Answer from the drawing. Dimensions are ordinates in mm from the lowest x, y and z of the part. A direction names the side the tool comes from. Give positions to 0.01 mm unless a question says otherwise; leave off trailing zeros. Loops run counter-clockwise (first coordinate to the right, second up) from the corner with the lowest first, then second, coordinate; pieces in that order, holes last. Notation, with made-up numbers: (4, -37.75) - (33, -37.75) arc R13 ccw to (33, -18.75) - close; hole circle Ø4 at (14, -35). An arc over 180 degrees is marked (long way). Put each result on its own line as item: value. Start each with the question number.
1. A cutting plane is placed at B-B, the plane y = 46.5. Determine the outline of the cut face in (x, z) (3 decimals), plus the area to 3 significant figures.
2. A cutting plane is placed at C-C, the plane z = 7. Determine the outline of the cut face in (x, y) (3 decimals).
3. A cutting plane is placed at A-A, the plane x = 41. Determine the outline of the cut face in (y, z), plus the area to 3 significant figures.
4. A cutting plane is placed at D-D, the plane x = 18.5. Determine the outline of the cut face in (y, z), plus the area to 3 significant figures.
5. For a pull along X with two mould halves and no side action, classify the marked faces 1, 2 and 3 as released by +X, released by -X, zero draft, split by the parting line, or undercut.
6. For the marked faces 4, 5, 6, 7 and 8, determine the directions among +Z, -Z, +X, -X, +Y, -Y from which every point of the face is accessible in a straight line to the end or side of a thin tool.
7. Consider L1, parallel to Z at x = 45.5, y = 50.5; L2, parallel to Y at x = 26, z = 29; L3, parallel to X at y = 46, z = 45 (3 decimals). Determine where each line is inside the solid, lowest interval first. Write a range as from..to.
8. Given pin 1 Ø11.5 at (x, y) = (20, 50.5) entering from +Z; pin 2 Ø5 at (y, z) = (46, 42) entering from -X (3 decimals); pin 3 Ø12 at (x, z) = (40, 19.5) entering from +Y; pin 4 Ø3 at (y, z) = (47.5, 43.5) entering from +X (3 decimals), each flat-ended and moving along its own axis, determine where each tip first touches the part or whether it passes through.
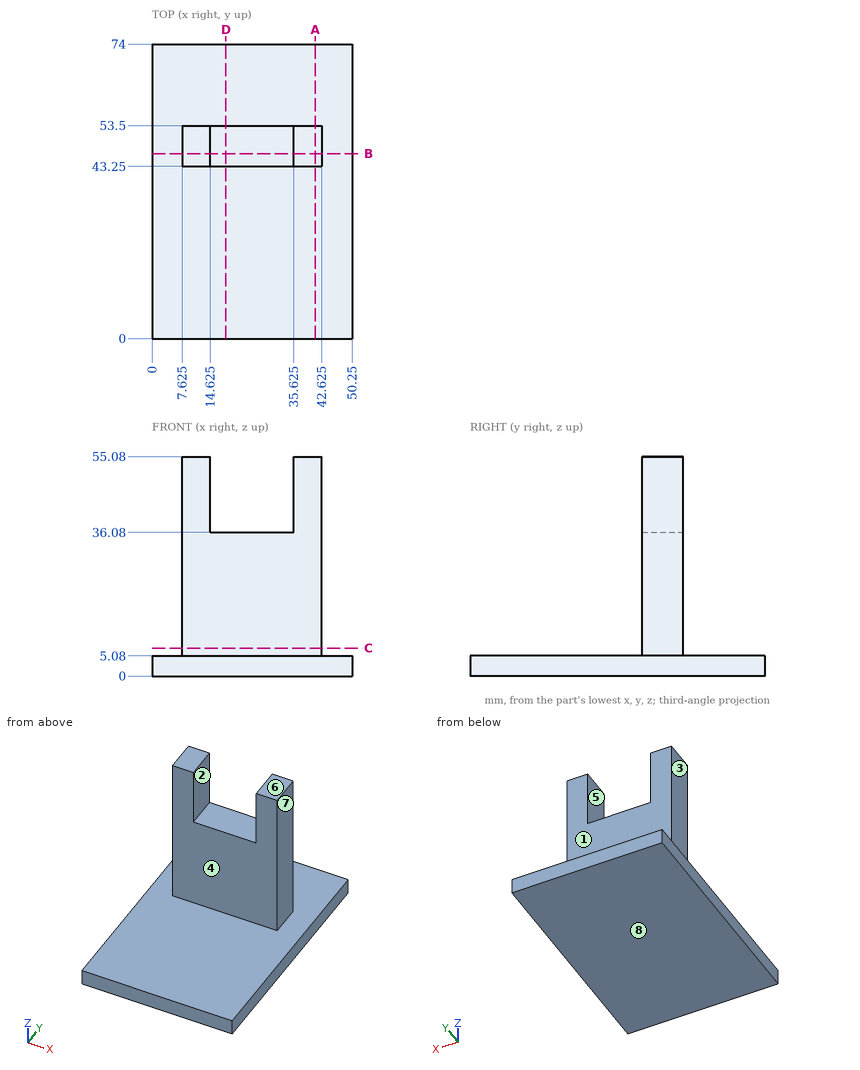
Return value:
1. outline: (0, 0) - (50.25, 0) - (50.25, 5.08) - (42.625, 5.08) - (42.625, 55.08) - (35.625, 55.08) - (35.625, 36.08) - (14.625, 36.08) - (14.625, 55.08) - (7.625, 55.08) - (7.625, 5.08) - (0, 5.08) - close
1. area: 1,610 mm2
2. outline: (7.625, 43.25) - (42.625, 43.25) - (42.625, 53.5) - (7.625, 53.5) - close
3. outline: (0, 0) - (74, 0) - (74, 5.08) - (53.5, 5.08) - (53.5, 55.08) - (43.25, 55.08) - (43.25, 5.08) - (0, 5.08) - close
3. area: 888 mm2
4. outline: (0, 0) - (74, 0) - (74, 5.08) - (53.5, 5.08) - (53.5, 36.08) - (43.25, 36.08) - (43.25, 5.08) - (0, 5.08) - close
4. area: 694 mm2
5. face 1: zero draft
5. face 2: undercut
5. face 3: released by -X
6. face 4: +Z, +X, -X, -Y
6. face 5: +Z, +Y, -Y
6. face 6: +Z, +X, -X, +Y, -Y
6. face 7: +Z, +X, +Y, -Y
6. face 8: -Z, +X, -X, +Y, -Y
7. L1: z = 0..5.08
7. L2: y = 43.25..53.5
7. L3: x = 7.625..14.625, 35.625..42.625
8. pin 1: stops at z = 55.08
8. pin 2: stops at x = 7.625
8. pin 3: stops at y = 53.5
8. pin 4: stops at x = 42.625
